For this review, take the finished solid that the model builds, in its own axes (mm). Face numbers are marked on the shaded views. A direction names the side the tool comes from. Give positions to 0.01 mm unless a question says otherwise; leave off trailing zeros. Loops run counter-clockwise (first coordinate to the right, second up) from the corner with the lowest first, then second, coordinate; pieces in that order, holes last. Notation, with made-up numbers: (65.5, -5) -> (87.5, -5) arc R31 cw to (87.5, 30) -> close; hole circle Ø3 at (57, 66.5). An arc over 180 degrees is marked (long way). One line per question, with ' | ' between items. Start each with the question number.
(1) Consider section B-B (y = 18.25). Write out the cut boundary in (x, z).
(2) Wall thickness on probe 1 along X at (y, z) = (9.5, 0); probe 2 along Z at (x, y) = (4, 12.5); probe 3 along X at (y, z) = (5.75, -11.5): over which ranges is each line inside the solid? List them lowest first.
(3) Insertion check: P1, Ø5.5, axis at x = 4.5, y = 19.5, coming from the -Z side; P2, Ø4, axis at y = 6.5, z = -14, coming from the +X side; P3, Ø1.5, axis at y = 12.5, z = 15, coming from the +X side. Each pin has a flat end and moves straight along its axis. Give the tip position at first contact, or say it passes through.
(4) Consider section A-A (x = 0). Write out the cut boundary in (y, z).
(5) Consider section D-D (y = 8). Write out the cut boundary in (x, z).
(6) Tool access review of the marked faces 4, 5 and 6: name each direction out of +Z, -Z, +X, -X, +Y, -Y from which nothing blocks a thin tool from reaching the whole face with its end or side.
(7) Consider section C-C (z = 5). Write out the cut boundary in (x, y).
(8) Draft analysis for pull direction Z (two halves, no side actions). For the marked faces 1, 2 and 3, state which applies: +Z half, -Z half, draft (parallel to the pull), parting line (faces both ways), or undercut.
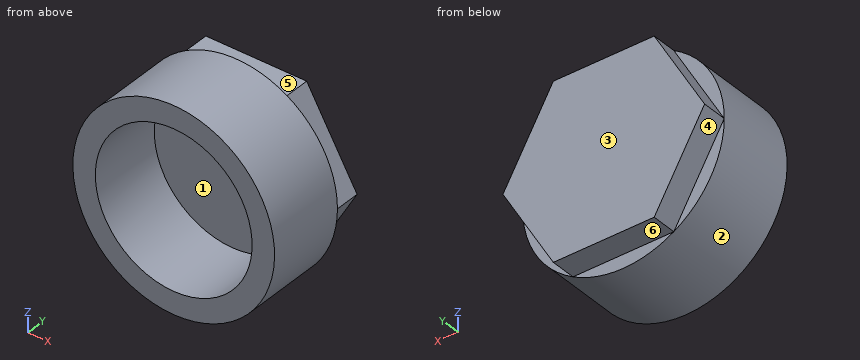
from build123d import *

# Parameters (mm, degrees)
TAGLIO_ESTRUSIONE1_START = -5
TAGLIO_ESTRUSIONE1_DEPTH = 5


with BuildPart() as part:
    # Schizzo1 → Rivoluzione1 (revolve)
    with BuildSketch(Plane.XY, mode=Mode.PRIVATE) as rivoluzione1_sk:
        Polygon((-15.5465, 0), (-15.5465, 15), (0, 15), (0, 21), (-20, 21), (-20, 0), align=None)
    revolve(rivoluzione1_sk.sketch.rotate(Axis((0, 0, 0), (0, 1, 0)), 270), axis=Axis((0, 0, 0), (0, 1, 0)))

    # Schizzo2 → Taglio-Estrusione1 (cut)
    with BuildSketch(Plane(origin=(0, 21, 0), x_dir=(1, 0, 0), z_dir=(0, 1, 0)).offset(TAGLIO_ESTRUSIONE1_START)):
        with BuildLine():
            Line((-20, 0), (-10, 17.320508076))
            ThreePointArc((-10, 17.320508076), (-17.320508076, 10), (-20, 0))
        make_face()
        with BuildLine():
            Line((-10, -17.320508076), (-20, 0))
            ThreePointArc((-20, 0), (-17.320508076, -10), (-10, -17.320508076))
        make_face()
        with BuildLine():
            Line((10, -17.320508076), (-10, -17.320508076))
            ThreePointArc((-10, -17.320508076), (0, -20), (10, -17.320508076))
        make_face()
        with BuildLine():
            ThreePointArc((10, -17.320508076), (17.320508076, -10), (20, 0))
            Line((20, 0), (10, -17.320508076))
        make_face()
        with BuildLine():
            ThreePointArc((20, 0), (17.320508076, 10), (10, 17.320508076))
            Line((10, 17.320508076), (20, 0))
        make_face()
        with BuildLine():
            ThreePointArc((10, 17.320508076), (0, 20), (-10, 17.320508076))
            Line((-10, 17.320508076), (10, 17.320508076))
        make_face()
    extrude(amount=TAGLIO_ESTRUSIONE1_DEPTH, mode=Mode.SUBTRACT)


solid = part.part
A:
1) outline: (-20, 0) -> (-10, -17.32) -> (10, -17.32) -> (20, 0) -> (10, 17.32) -> (-10, 17.32) -> close
2) probe 1: x = -20 to -15.55, 15.55 to 20 | probe 2: z = -19.6 to -15.02, 15.02 to 19.6 | probe 3: x = -16.36 to -10.46, 10.46 to 16.36
3) P1: stops at z = -17.32 | P2: stops at x = 16 | P3: stops at x = 14.03
4) outline: (0, -20) -> (16, -20) -> (16, -17.32) -> (21, -17.32) -> (21, 17.32) -> (16, 17.32) -> (16, 20) -> (0, 20) -> (0, 15.55) -> (15, 15.55) -> (15, -15.55) -> (0, -15.55) -> close
5) outline: circle Ø40 at (0, 0); hole circle Ø31.09 at (0, 0)
6) face 4: -Z, -X, +Y | face 5: +Z, +X, -X, +Y | face 6: -Z, +X, -X, +Y
7) outline: (-19.36, 0) -> (-14.72, 0) -> (-14.72, 15) -> (14.72, 15) -> (14.72, 0) -> (19.36, 0) -> (19.36, 16) -> (17.11, 16) -> (17.11, 21) -> (-17.11, 21) -> (-17.11, 16) -> (-19.36, 16) -> close
8) face 1: undercut | face 2: parting line | face 3: draft
